from build123d import *

# Parameters (mm, degrees)
F1_DEPTH = 25.4
F2_W     = 50.8
F2_H     = 25.4
F3_DEPTH = 25.4
F5_DEPTH = 25.4


with BuildPart() as f1:
    # F0 (on Top) → F1 (new body)
    with BuildSketch(Plane.XY):
        with BuildLine():
            Line((-60.40253, 55.21483), (-60.424231, 55.21483))
            Line((-60.424231, 55.21483), (-60.424231, -33.68517))
            Line((-60.424231, -33.68517), (-9.624231, -33.68517))
            Line((-9.624231, -33.68517), (-9.624231, 55.21483))
            Line((-9.624231, 55.21483), (-9.645933, 55.21483))
            ThreePointArc((-9.645933, 55.21483), (-35.024231, 80.593129), (-60.40253, 55.21483))
        make_face()
    extrude(amount=F1_DEPTH)

    # F2 (on face) → F3 (join)
    with BuildSketch(Plane.XY.offset(25.4)):
        with Locations((-35.024231, -20.98517)):
            Rectangle(F2_W, F2_H)
    extrude(amount=F3_DEPTH)

    # F4 (on face) → F5 (cut)
    with BuildSketch(Plane.XY.offset(25.4)):
        with BuildLine():
            Line((-35.024231, 17.11483), (-22.324231, 17.11483))
            ThreePointArc((-22.324231, 17.11483), (-26.043975, 26.095086), (-35.024231, 29.81483))
            Line((-35.024231, 29.81483), (-35.024231, 17.11483))
        make_face()
        with BuildLine():
            ThreePointArc((-35.024231, 4.41483), (-26.043975, 8.134574), (-22.324231, 17.11483))
            Line((-22.324231, 17.11483), (-35.024231, 17.11483))
            Line((-35.024231, 17.11483), (-35.024231, 4.41483))
        make_face()
        with BuildLine():
            Line((-35.024231, 17.11483), (-35.024231, 29.81483))
            ThreePointArc((-35.024231, 29.81483), (-44.004487, 26.095086), (-47.724231, 17.11483))
            Line((-47.724231, 17.11483), (-35.024231, 17.11483))
        make_face()
        with BuildLine():
            ThreePointArc((-47.724231, 17.11483), (-44.004487, 8.134574), (-35.024231, 4.41483))
            Line((-35.024231, 4.41483), (-35.024231, 17.11483))
            Line((-35.024231, 17.11483), (-47.724231, 17.11483))
        make_face()
        with BuildLine():
            Line((-35.024231, 55.203979), (-22.335082, 55.203979))
            ThreePointArc((-22.335082, 55.203979), (-26.051648, 64.176563), (-35.024231, 67.893129))
            Line((-35.024231, 67.893129), (-35.024231, 55.203979))
        make_face()
        with BuildLine():
            ThreePointArc((-35.024231, 42.51483), (-26.051648, 46.231396), (-22.335082, 55.203979))
            Line((-22.335082, 55.203979), (-35.024231, 55.203979))
            Line((-35.024231, 55.203979), (-35.024231, 42.51483))
        make_face()
        with BuildLine():
            Line((-35.024231, 55.203979), (-35.024231, 67.893129))
            ThreePointArc((-35.024231, 67.893129), (-43.996815, 64.176563), (-47.713381, 55.203979))
            Line((-47.713381, 55.203979), (-35.024231, 55.203979))
        make_face()
        with BuildLine():
            ThreePointArc((-47.713381, 55.203979), (-43.996815, 46.231396), (-35.024231, 42.51483))
            Line((-35.024231, 42.51483), (-35.024231, 55.203979))
            Line((-35.024231, 55.203979), (-47.713381, 55.203979))
        make_face()
    extrude(amount=-F5_DEPTH, mode=Mode.SUBTRACT)


solid = f1.part
Build history of the part. All positions in model axes, mm. A direction names the side the tool comes from. Round coordinates to 2 decimals unless told otherwise and drop trailing zeros. Write each loop counter-clockwise with the first axis right and the second up, starting at its lowest first coordinate (ties: lowest second). Pieces come first, ordered by that corner, then holes. Notation, with made-up numbers: (-7, 2.25) -> (23, 2.25) arc R24 ccw to (23, 32.25) -> close; hole circle Ø3 at (61.5, -23.75). An arc over 180 degrees is marked (long way). Write item = value, one per line.
(1) Band-saw the part on B-B (x = -33). Give the cut face in (y, z).
Answer:
outline = (-33.69, 0) -> (4.58, 0) -> (4.58, 25.4) -> (-8.29, 25.4) -> (-8.29, 50.8) -> (-33.69, 50.8) -> close; (29.65, 0) -> (42.68, 0) -> (42.68, 25.4) -> (29.65, 25.4) -> close; (67.73, 0) -> (80.51, 0) -> (80.51, 25.4) -> (67.73, 25.4) -> close
(2) Tool access for faces 1 (the face through (-35, -8.285, 38)), 2 (the face through (-34.466, 80.587, 12.522)): list every direction of +Z, -Z, +X, -X, +Y, -Y with a clear straight run to the whole face (end or side of a thin tool).
Answer:
face_1 = +Z, +X, -X, +Y
face_2 = +Z, -Z, +Y
(3) Probe L1, parallel to Y at x = -39.5, z = 23; L2, parallel to Z at x = -23, y = 48; L3, parallel to Y at x = -25, z = 20.5. List the from-to ranges inside material, lowest first.
Answer:
L1 = -33.69 to 5.23, 29 to 43.33, 67.08 to 80.2
L2 = 0 to 25.4
L3 = -33.69 to 9.32, 24.91 to 47.42, 62.98 to 78.53
(4) Flat gauge pins, fed straight in: pin 1 (6 mm diameter, centred on x = -40.5, y = 68.5, fed in from +Z); pin 2 (20.5 mm diameter, centred on x = -38.5, z = 43, fed in from +Y); pin 3 (4 mm diameter, centred on x = -39, z = 24, fed in from +Y). Where does each tip first touch, or does it go through?
Answer:
pin_1 = 25.4
pin_2 = -8.29
pin_3 = 80.52
(5) Band-saw the part on A-A (z = 7.5). State how many separate pieces and enclosed holes the cut face has, then the cut area to 3 significant figures.
Answer:
separate_pieces = 1
enclosed_holes = 2
area = 4,520 mm2
(6) Band-saw the part on D-D (y = -6). Give the cut face in (x, z), then the cut area to 3 significant figures.
Answer:
outline = (-60.42, 0) -> (-9.62, 0) -> (-9.62, 25.4) -> (-60.42, 25.4) -> close
area = 1,290 mm2
(7) Band-saw the part on C-C (y = 54). Give the cut face in (x, z).
Answer:
outline = (-60.42, 0) -> (-47.66, 0) -> (-47.66, 25.4) -> (-60.42, 25.4) -> close; (-22.39, 0) -> (-9.62, 0) -> (-9.62, 25.4) -> (-22.39, 25.4) -> close
